Here's how the part is built. I have some questions about the finished solid (model axes, mm). A direction names the side the tool comes from. Give positions to 0.01 mm unless a question says otherwise; leave off trailing zeros. Loops run counter-clockwise (first coordinate to the right, second up) from the corner with the lowest first, then second, coordinate; pieces in that order, holes last.
Q1. Suppose I cut it at B-B (x = 1.5). List the corners of the cut face in (y, z) for me, and give its area (3 significant figures).
Q2. I need wall thicknesses on probe 1 along X at (y, z) = (0, -3.5); probe 2 along X at (y, z) = (1.5, -2); probe 3 along Y at (x, z) = (1, -3). Which ranges of each line are inside material? Lowest first, please.
Q3. Thinking about a two-plate mould opening in X: for faces 1 (the face through (5, -0.84, -4)), 2 (the face through (-6.2, -0.1, -3.9)), 3 (the face through (0, 0, -8)), 4 (the face through (1.4, 0.84, -3.9)), which applies, pulls with the +X half, pulls with the -X half, needs draft (parallel to the pull), parting line crosses it, or undercut?
Q4. Suppose I cut it at A-A (y = 0). List the corners of the cut face in (x, z) for me.
Q5. For faces 5 (the face through (6.2, 0.1, -3.9)), 6 (the face through (-5, -0.84, -4)), which set-ups out of +Z, -Z, +X, -X, +Y, -Y let a thin tool reach every point of the face, with its end or its side?
Q6. I'm going to push flat-ended pins straight in: P1, Ø0.5, axis at x = 5, z = -2.5, coming from the -Y side; P2, Ø1, axis at y = -1.5, z = -3, coming from the -X side; P3, Ø1, axis at x = -5, z = -3, coming from the -Y side. Where does each tip first touch, or does it pass through?
Q7. Suppose I cut it at C-C (y = 1). List the corners of the cut face in (x, z) for me, and give its area (3 significant figures).
Q8. Suppose I cut it at D-D (z = -2.5). Count the separate pieces of the cut face and the enclosed holes in it, and give its area (3 significant figures).
```python
from build123d import *

# Parameters (mm, degrees)
BOSS_EXTRUDE1_DEPTH   = 8
CUT_EXTRUDE1_DEPTH    = 11.585367259
FILLET1_R             = 0.4
FILLET2_R             = 0.4
FILLET3_R             = 0.4
FILLET4_R             = 0.4
FILLET5_R             = 0.1
FILLET6_R             = 0.1
FILLET7_R             = 0.1
FILLET8_R             = 0.1
FILLET9_R             = 0.1
FILLET10_R            = 0.1
FILLET11_R            = 0.1
FILLET12_R            = 0.1
FILLET1_OF_MIRROR1_R  = 0.4
FILLET2_OF_MIRROR1_R  = 0.4
FILLET3_OF_MIRROR1_R  = 0.4
FILLET4_OF_MIRROR1_R  = 0.4
FILLET5_OF_MIRROR1_R  = 0.1
FILLET6_OF_MIRROR1_R  = 0.1
FILLET7_OF_MIRROR1_R  = 0.1
FILLET8_OF_MIRROR1_R  = 0.1
FILLET9_OF_MIRROR1_R  = 0.1
FILLET10_OF_MIRROR1_R = 0.1
FILLET11_OF_MIRROR1_R = 0.1
FILLET12_OF_MIRROR1_R = 0.1


with BuildPart() as part:
    # Sketch2 → Boss-Extrude1 (new body)
    with BuildSketch(Plane.XY):
        with BuildLine():
            Line((-3.1, 3.1), (3.1, 3.1))
            ThreePointArc((3.1, 3.1), (6.2, 0), (3.1, -3.1))
            Line((3.1, -3.1), (-3.1, -3.1))
            ThreePointArc((-3.1, -3.1), (-6.2, 0), (-3.1, 3.1))
        make_face()
    extrude(amount=-BOSS_EXTRUDE1_DEPTH)

    # Sketch4 → Cut-Extrude1 (cut, through all)
    with BuildSketch(Plane.XY):
        with BuildLine():
            Line((-3.94, -0.84), (-3.94, -2.248199279))
            ThreePointArc((-3.94, -2.248199279), (-3.1, -2.4), (-2.26, -2.248199279))
            Line((-2.26, -2.248199279), (-2.26, -0.84))
            Line((-2.26, -0.84), (-0.851800721, -0.84))
            ThreePointArc((-0.851800721, -0.84), (-0.7, 0), (-0.851800721, 0.84))
            Line((-0.851800721, 0.84), (-2.26, 0.84))
            Line((-2.26, 0.84), (-2.26, 2.248199279))
            ThreePointArc((-2.26, 2.248199279), (-3.1, 2.4), (-3.94, 2.248199279))
            Line((-3.94, 2.248199279), (-3.94, 0.84))
            Line((-3.94, 0.84), (-5.348199279, 0.84))
            ThreePointArc((-5.348199279, 0.84), (-5.5, 0), (-5.348199279, -0.84))
            Line((-5.348199279, -0.84), (-3.94, -0.84))
        make_face()
    cut_extrude1 = extrude(amount=-CUT_EXTRUDE1_DEPTH, mode=Mode.SUBTRACT)

    # Fillet1
    fillet1_edges = [part.edges().sort_by_distance(p)[0] for p in [
        (-3.94, -0.84, -4),
    ]]
    fillet(fillet1_edges, radius=FILLET1_R)

    # Fillet2
    fillet2_edges = [part.edges().sort_by_distance(p)[0] for p in [
        (-3.94, 0.84, -4),
    ]]
    fillet(fillet2_edges, radius=FILLET2_R)

    # Fillet3
    fillet3_edges = [part.edges().sort_by_distance(p)[0] for p in [
        (-2.26, 0.84, -4),
    ]]
    fillet(fillet3_edges, radius=FILLET3_R)

    # Fillet4
    fillet4_edges = [part.edges().sort_by_distance(p)[0] for p in [
        (-2.26, -0.84, -4),
    ]]
    fillet(fillet4_edges, radius=FILLET4_R)

    # Fillet5
    fillet5_edges = [part.edges().sort_by_distance(p)[0] for p in [
        (-3.94, -2.248199279, -4),
    ]]
    fillet(fillet5_edges, radius=FILLET5_R)

    # Fillet6
    fillet6_edges = [part.edges().sort_by_distance(p)[0] for p in [
        (-2.26, -2.248199279, -4),
    ]]
    fillet(fillet6_edges, radius=FILLET6_R)

    # Fillet7
    fillet7_edges = [part.edges().sort_by_distance(p)[0] for p in [
        (-0.851800721, 0.84, -4),
    ]]
    fillet(fillet7_edges, radius=FILLET7_R)

    # Fillet8
    fillet8_edges = [part.edges().sort_by_distance(p)[0] for p in [
        (-0.851800721, -0.84, -4),
    ]]
    fillet(fillet8_edges, radius=FILLET8_R)

    # Fillet9
    fillet9_edges = [part.edges().sort_by_distance(p)[0] for p in [
        (-2.26, 2.248199279, -4),
    ]]
    fillet(fillet9_edges, radius=FILLET9_R)

    # Fillet10
    fillet10_edges = [part.edges().sort_by_distance(p)[0] for p in [
        (-3.94, 2.248199279, -4),
    ]]
    fillet(fillet10_edges, radius=FILLET10_R)

    # Fillet11
    fillet11_edges = [part.edges().sort_by_distance(p)[0] for p in [
        (-5.348199279, 0.84, -4),
    ]]
    fillet(fillet11_edges, radius=FILLET11_R)

    # Fillet12
    fillet12_edges = [part.edges().sort_by_distance(p)[0] for p in [
        (-5.348199279, -0.84, -4),
    ]]
    fillet(fillet12_edges, radius=FILLET12_R)

    # Mirror1: Cut-Extrude1 across plane
    add(cut_extrude1.mirror(Plane(origin=(0, 0, 0), x_dir=(0, 0, 1), z_dir=(1, 0, 0))), mode=Mode.SUBTRACT)

    # Fillet1 of Mirror1
    fillet1_of_mirror1_edges = [part.edges().sort_by_distance(p)[0] for p in [
        (3.94, -0.84, -4),
    ]]
    fillet(fillet1_of_mirror1_edges, radius=FILLET1_OF_MIRROR1_R)

    # Fillet2 of Mirror1
    fillet2_of_mirror1_edges = [part.edges().sort_by_distance(p)[0] for p in [
        (3.94, 0.84, -4),
    ]]
    fillet(fillet2_of_mirror1_edges, radius=FILLET2_OF_MIRROR1_R)

    # Fillet3 of Mirror1
    fillet3_of_mirror1_edges = [part.edges().sort_by_distance(p)[0] for p in [
        (2.26, 0.84, -4),
    ]]
    fillet(fillet3_of_mirror1_edges, radius=FILLET3_OF_MIRROR1_R)

    # Fillet4 of Mirror1
    fillet4_of_mirror1_edges = [part.edges().sort_by_distance(p)[0] for p in [
        (2.26, -0.84, -4),
    ]]
    fillet(fillet4_of_mirror1_edges, radius=FILLET4_OF_MIRROR1_R)

    # Fillet5 of Mirror1
    fillet5_of_mirror1_edges = [part.edges().sort_by_distance(p)[0] for p in [
        (3.94, -2.248199279, -4),
    ]]
    fillet(fillet5_of_mirror1_edges, radius=FILLET5_OF_MIRROR1_R)

    # Fillet6 of Mirror1
    fillet6_of_mirror1_edges = [part.edges().sort_by_distance(p)[0] for p in [
        (2.26, -2.248199279, -4),
    ]]
    fillet(fillet6_of_mirror1_edges, radius=FILLET6_OF_MIRROR1_R)

    # Fillet7 of Mirror1
    fillet7_of_mirror1_edges = [part.edges().sort_by_distance(p)[0] for p in [
        (0.851800721, 0.84, -4),
    ]]
    fillet(fillet7_of_mirror1_edges, radius=FILLET7_OF_MIRROR1_R)

    # Fillet8 of Mirror1
    fillet8_of_mirror1_edges = [part.edges().sort_by_distance(p)[0] for p in [
        (0.851800721, -0.84, -4),
    ]]
    fillet(fillet8_of_mirror1_edges, radius=FILLET8_OF_MIRROR1_R)

    # Fillet9 of Mirror1
    fillet9_of_mirror1_edges = [part.edges().sort_by_distance(p)[0] for p in [
        (2.26, 2.248199279, -4),
    ]]
    fillet(fillet9_of_mirror1_edges, radius=FILLET9_OF_MIRROR1_R)

    # Fillet10 of Mirror1
    fillet10_of_mirror1_edges = [part.edges().sort_by_distance(p)[0] for p in [
        (3.94, 2.248199279, -4),
    ]]
    fillet(fillet10_of_mirror1_edges, radius=FILLET10_OF_MIRROR1_R)

    # Fillet11 of Mirror1
    fillet11_of_mirror1_edges = [part.edges().sort_by_distance(p)[0] for p in [
        (5.348199279, 0.84, -4),
    ]]
    fillet(fillet11_of_mirror1_edges, radius=FILLET11_OF_MIRROR1_R)

    # Fillet12 of Mirror1
    fillet12_of_mirror1_edges = [part.edges().sort_by_distance(p)[0] for p in [
        (5.348199279, -0.84, -4),
    ]]
    fillet(fillet12_of_mirror1_edges, radius=FILLET12_OF_MIRROR1_R)


solid = part.part
```
Solutions:
1. outline: (-3.1, -8) - (-0.84, -8) - (-0.84, 0) - (-3.1, 0) - close; (0.84, -8) - (3.1, -8) - (3.1, 0) - (0.84, 0) - close
1. area: 36.2 mm2
2. probe 1: x = -6.2 to -5.5, -0.7 to 0.7, 5.5 to 6.2
2. probe 2: x = -5.81 to -3.94, -2.26 to 2.26, 3.94 to 5.81
2. probe 3: y = -3.1 to -0.84, 0.84 to 3.1
3. face 1: undercut
3. face 2: pulls with the -X half
3. face 3: needs draft
3. face 4: undercut
4. outline: (-6.2, -8) - (-5.5, -8) - (-5.5, 0) - (-6.2, 0) - close; (-0.7, -8) - (0.7, -8) - (0.7, 0) - (-0.7, 0) - close; (5.5, -8) - (6.2, -8) - (6.2, 0) - (5.5, 0) - close
5. face 5: +Z, -Z, +X
5. face 6: +Z, -Z
6. P1: stops at y = -2.62
6. P2: stops at x = -6.03
6. P3: stops at y = -2.77
7. outline: (-6.03, -8) - (-4.02, -8) - (-4.02, 0) - (-6.03, 0) - close; (-2.18, -8) - (2.18, -8) - (2.18, 0) - (-2.18, 0) - close; (4.02, -8) - (6.03, -8) - (6.03, 0) - (4.02, 0) - close
7. area: 67.1 mm2
8. separate pieces: 1
8. enclosed holes: 2
8. area: 42.4 mm2
